Design review of the part built by this model. Coordinates are the model's own, in mm. Coordinates: 2 decimals unless noted, no trailing zeros. Write each loop counter-clockwise with the first axis right and the second up, starting at its lowest first coordinate (ties: lowest second). Pieces come first, ordered by that corner, then holes. Notation, with made-up numbers: (15, 57) - (31, 57) arc R8 ccw to (31, 71) - close; hole circle Ø4 at (0.5, 89.5). An arc over 180 degrees is marked (long way). One line per item, written item: value.
from build123d import *

# Parameters (mm, degrees)
F0_R     = 3
F1_DEPTH = 3


with BuildPart() as f1:
    # F0 (on Right) → F1 (new body)
    with BuildSketch(Plane.YZ):
        with BuildLine():
            ThreePointArc((5, 0), (0, 5), (-5, 0))
            Line((-5, 0), (-5, -45))
            ThreePointArc((-5, -45), (0, -50), (5, -45))
            Line((5, -45), (5, 0))
        make_face()
        with Locations((0, -45)):
            Circle(F0_R, mode=Mode.SUBTRACT)
        Circle(F0_R, mode=Mode.SUBTRACT)
    extrude(amount=F1_DEPTH)


solid = f1.part
1. Wall thickness on line 1 along Z through (x, y) = (2.1, 0); line 2 along Z through (x, y) = (1.55, 1.75); line 3 along Y through (x, z) = (2.85, -2.5): over which ranges is each line inside the solid? List them lowest first.
Answer block:
line 1: z = -50 to -48, -42 to -3, 3 to 5
line 2: z = -49.68 to -47.44, -42.56 to -2.44, 2.44 to 4.68
line 3: y = -5 to -1.66, 1.66 to 5
2. Consider section B-B, the plane z = -45.5. Write out the cut boundary in (x, y), then the cut area to 3 significant figures.
Answer block:
outline: (0, -4.97) - (3, -4.97) - (3, -2.96) - (0, -2.96) - close; (0, 2.96) - (3, 2.96) - (3, 4.97) - (0, 4.97) - close
area: 12.1 mm^2
3. Consider section D-D, the plane y = 2. Write out the cut boundary in (x, z), then the cut area to 3 significant figures.
Answer block:
outline: (0, -49.58) - (3, -49.58) - (3, -47.24) - (0, -47.24) - close; (0, -42.76) - (3, -42.76) - (3, -2.24) - (0, -2.24) - close; (0, 2.24) - (3, 2.24) - (3, 4.58) - (0, 4.58) - close
area: 136 mm^2
4. Mouldability with a two-part tool opening along Z and no side actions: class faces 1 (the face through (1, -5, -22)), 2 (the face through (1, -3, 0)), 3 (the face through (1, 0, -50)) as released by +Z, released by -Z, zero draft, split by the parting line, or undercut.
Answer block:
face 1: zero draft
face 2: undercut
face 3: released by -Z
5. Consider section A-A, the plane y = 0. Write out the cut boundary in (x, z).
Answer block:
outline: (0, -50) - (3, -50) - (3, -48) - (0, -48) - close; (0, -42) - (3, -42) - (3, -3) - (0, -3) - close; (0, 3) - (3, 3) - (3, 5) - (0, 5) - close
6. Consider section C-C, the plane x = 0.5. Write out the cut boundary in (y, z).
Answer block:
outline: (-5, -45) arc R5 ccw to (5, -45) - (5, 0) arc R5 ccw to (-5, 0) - close; hole circle Ø6 at (0, -45); hole circle Ø6 at (0, 0)
